Here's how the part is built. I have some questions about the finished solid (model axes, mm). Give positions to 0.01 mm unless a question says otherwise; leave off trailing zeros. Loops run counter-clockwise (first coordinate to the right, second up) from the corner with the lowest first, then second, coordinate; pieces in that order, holes last. Notation, with made-up numbers: (-32, 80) - (2, 80) arc R3 cw to (2, 84) - close; hole circle Ø7 at (49, 53.5). An arc over 180 degrees is marked (long way). Use one line per item in the form item = value.
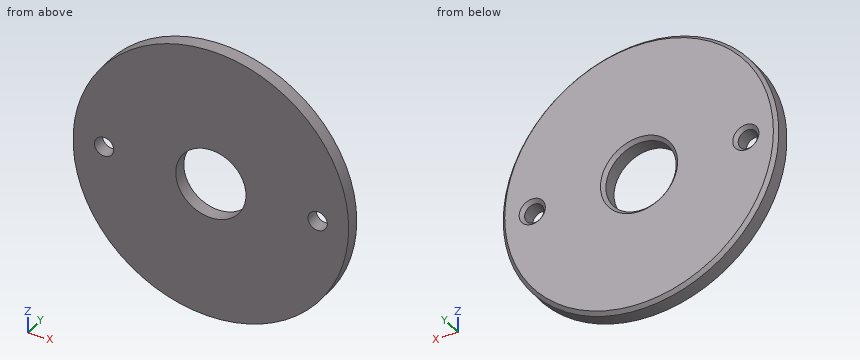
from build123d import *

# Parameters (mm, degrees)
SKETCH1_R           = 50.8
SKETCH1_R_2         = 3.556
SKETCH1_R_3         = 12.954
BOSS_EXTRUDE1_DEPTH = 6.35
CHAMFER1_SIZE       = 1.27


with BuildPart() as part:
    # Sketch1 → Boss-Extrude1 (new body)
    with BuildSketch(Plane(origin=(0, 0, 0), x_dir=(1, 0, 0), z_dir=(0, 1, 0))):
        Circle(SKETCH1_R)
        with Locations((-39.37, -0.992258715)):
            Circle(SKETCH1_R_2, mode=Mode.SUBTRACT)
        Circle(SKETCH1_R_3, mode=Mode.SUBTRACT)
        with Locations((39.37, 0.992258715)):
            Circle(SKETCH1_R_2, mode=Mode.SUBTRACT)
    extrude(amount=BOSS_EXTRUDE1_DEPTH)

    # Chamfer1
    chamfer1_edges = [part.edges().sort_by_distance(p)[0] for p in [
        (35.814, 6.35, -0.992258715),
        (-50.8, 6.35, 0),
        (-42.926, 6.35, 0.992258715),
        (-12.954, 6.35, 0),
    ]]
    chamfer(chamfer1_edges, length=CHAMFER1_SIZE)


solid = part.part
(1) If we section it at B-B (y = 1.5): List the corners of the cut face in (x, z) for me, plus the area to 3 significant figures.
Geometry says:
outline = circle Ø101.6 at (0, 0); hole circle Ø7.11 at (-39.37, 0.99); hole circle Ø25.91 at (0, 0); hole circle Ø7.11 at (39.37, -0.99)
area = 7,500 mm²
(2) If I drill on probe 1 along X at (y, z) = (4.5, 4); probe 2 along Z at (x, y) = (0, 2.65); probe 3 along X at (y, z) = (3.45, 0), over which ranges is the centre line in solid material (lowest first)?
Geometry says:
probe_1 = -50.64 to -41.27, -37.47 to -12.32, 12.32 to 50.64
probe_2 = -50.8 to -12.95, 12.95 to 50.8
probe_3 = -50.8 to -42.78, -35.96 to -12.95, 12.95 to 35.96, 42.78 to 50.8
(3) If we section it at A-A (x = 0): List the corners of the cut face in (y, z) for me, plus the area to 3 significant figures.
Geometry says:
outline = (0, -50.8) - (5.08, -50.8) - (6.35, -49.53) - (6.35, -14.22) - (5.08, -12.95) - (0, -12.95) - close; (0, 12.95) - (5.08, 12.95) - (6.35, 14.22) - (6.35, 49.53) - (5.08, 50.8) - (0, 50.8) - close
area = 477 mm²
(4) For P1, Ø3, axis at x = 9.5, y = 5, coming from the -Z side; P2, Ø1, axis at y = 2, z = -9, coming from the -X side; P3, Ø8, axis at x = -39.37, z = 0.99, coming from the -Y side; P4, Ø1, axis at y = 5.5, z = 22.5, coming from the -X side, each with a flat end and sliding along its axis, tell me the tip position at first contact or that it passes through.
Geometry says:
P1 = -50.17
P2 = -50.08
P3 = 0
P4 = -45.68
